Autodesk Fusion 360 part; units mm, degrees
sketch "Sketch1" plane through (0, 0, 0) normal (1, 0, 0) x (0, 1, 0)
  line L0 (0, 7) -> (2, 7)
  line L1 (2, 7) -> (2, 0)
  line L2 (0, 0) -> (0, 12.5)
  line L3 (0, 12.5) -> (-30.8, 12.5)
  line L4 (-30.8, 12.5) -> (-30.8, 0)
  line L5 (-30.8, 12.2) -> (-61.6, 12.2)
  line L6 (-61.6, 12.2) -> (-61.6, 0)
  line L7 (-61.6, 0) -> (0, 0)
  line L8 (2, 3) -> (15, 3)
  line L9 (15, 3) -> (15, 0)
  line L10 (15, 0) -> (0, 0)
  line L11 (-61.6, -12.2) -> (-61.6, 0)
  line L12 (-30.8, -12.2) -> (-61.6, -12.2)
  line L13 (-30.8, -12.5) -> (-30.8, 0)
  line L14 (0, -12.5) -> (-30.8, -12.5)
  line L15 (0, 0) -> (0, -12.5)
  line L16 (0, -7) -> (2, -7)
  line L17 (2, -7) -> (2, 0)
  line L18 (2, -3) -> (15, -3)
  line L19 (15, -3) -> (15, 0)
  dimension "d1" = 25
  dimension "d2" = 24.4
  dimension "d3" = 14
  dimension "d4" = 6
  dimension "d5" = 15
  dimension "d7" = 30.8
  dimension "d8" = 30.8
  dimension "d9" = 2
revolve "Revolve1" add sketch "Sketch1" angle 360 about axis through (0, 1.75, 0) along (0, 1, 0) contours L0 L1 L2 L10 | L2 L3 L4 L7 | L1 L8 L9 L10 | L4 L5 L6 L7
sketch "Sketch2" plane through (0, 15, 0) normal (0, 1, 0) x (-1, 0, 0)
  circle A0 centre (0, 0) radius 3
  circle A1 centre (0, 0) radius 3
  line L0 (-2.2361, 2) -> (2.2361, 2)
  line L1 (0, 0) -> (0, -3)
  point P0 (0, -3)
  dimension "d11" = 6
  dimension "d12" = 5
extrude "Extrude1" cut sketch "Sketch2" against normal blind 9 contours A0 A1 L0 picked at (-0.1433, 0.3437)
sketch "Sketch3" plane through (0, 0, 0) normal (0, 1, 0) x (-1, 0, 0)
  circle A0 centre (0, 0) radius 12.5
  circle A1 centre (0, 0) radius 7
  circle A2 centre (-6.8943, 6.8943) radius 1.5
  circle A3 centre (6.8943, 6.8943) radius 1.5
  circle A4 centre (6.8943, -6.8943) radius 1.5
  circle A5 centre (-6.8943, -6.8943) radius 1.5
  line L0 (0, 0) -> (-6.8943, 6.8943)
  line L1 (0, 0) -> (6.8943, 6.8943)
  line L2 (6.8943, -6.8943) -> (0, 0)
  line L3 (0, 0) -> (-6.8943, -6.8943)
  circle A6 centre (0, 0) radius 9.75
  line L4 (0, 0) -> (2.2693, 0)
  dimension "d15" = 3
  dimension "d16" = 19.5
  dimension "d20" = 45
extrude "Extrude2" cut sketch "Sketch3" against normal blind 4.6 contours A3 L1 A6 | A3 L1 A6 | A4 L2 A6 | A4 L2 A6 | A2 L0 A6 | A2 L0 A6 | A3 A6 | A5 L3 A6 | A5 L3 A6 | A4 A6 | A2 A6 | A5 A6
sketch "Sketch4" plane through (0, -61.6, 0) normal (0, -1, 0) x (1, 0, 0)
  circle A0 centre (0, 0) radius 12.2
  circle A1 centre (0, 0) radius 10
  dimension "d23" = 20
extrude "Extrude3" add sketch "Sketch4" along normal blind 5 contours A1
extrude "Extrude4" add 1 faces at (-0.4082, 15, 2.4414) along direction (0, 1, 0) blind 5
equation "d16 = 14 mm + ( ( 25 - 14 ) / 2 ) * 1 mm"
Build history of the part. All positions in model axes, mm. A direction names the side the tool comes from. Give positions to 0.01 mm unless a question says otherwise; leave off trailing zeros. Order: outer loops, then holes, each group sorted by start corner. A loop starts at its lowest first (then second) coordinate and runs counter-clockwise, first axis right, second up. Notation, with made-up numbers: M 78,28.5 L 134,28.5 A14 cw 134,39.5 Z; hole C 48.25,82.5 d4. An arc over 180 degrees is marked long. Put each result on its own line as item: value.
Item 1: Wall check: probe 1 along Y at (x, z) = (7.5, 6.75); probe 2 along Y at (x, z) = (1.5, 4.5); probe 3 along X at (y, z) = (-15, 0). Give the ranges that are in metal, low to high.
Results are:
probe 1: -61.6 to -4.6
probe 2: -66.6 to 2
probe 3: -12.5 to 12.5
Item 2: Cut at C-C on y = -35. Write the cut outline in (x, z), then the cut area to 3 significant figures.
Results are:
outline: C 0,0 d24.4
area: 468 mm2
Item 3: Which spindle directions (+Z, -Z, +X, -X, +Y, -Y) get a long thin tool onto all of the face, cutting with end or side? Do faces 1 (the face through (7, -4.6, -7)), 2 (the face through (-0.54, -46.42, -12.19)), 3 (the face through (0, 6, 0)). Say none if no direction does.
Results are:
face 1: +Y
face 2: -Y
face 3: -Z, +X, -X, +Y
Item 4: Drop flat-ended pins along their axis: pin 1 Ø2.5 at (x, z) = (1, 0) entering from +Y; pin 2 Ø10 at (y, z) = (7, 7.5) entering from -X; pin 3 Ø3.5 at (x, z) = (6.89, 6.89) entering from +Y. Give the stop position or say it passes through.
Results are:
pin 1: y = 6
pin 2: x = -1.66
pin 3: y = 0
Item 5: Pull direction Z, two halves, no side cores. Call faces 4 (the face through (-5.4, 0, 5.4)), 5 (the face through (8.1, -2.3, 6)), 6 (the face through (0, 13, 2)), 7 (the face through (-7, -4.6, -7)): +Z half, -Z half, draft (parallel to the pull), parting line (faces both ways), or undercut.
Results are:
face 4: draft
face 5: undercut
face 6: -Z half
face 7: undercut
Item 6: Cut at B-B on x = 0. Write the cut outline in (y, z), then the cut area to 3 significant figures.
Results are:
outline: M -66.6,-10 L -61.6,-10 L -61.6,-12.2 L -30.8,-12.2 L -30.8,-12.5 L 0,-12.5 L 0,-7 L 2,-7 L 2,-3 L 6,-3 L 6,2 L 20,2 L 20,3 L 2,3 L 2,7 L 0,7 L 0,12.5 L -30.8,12.5 L -30.8,12.2 L -61.6,12.2 L -61.6,10 L -66.6,10 Z
area: 1,690 mm2
Item 7: Cut at A-A on z = 0. Write the cut outline in (x, y).
Results are:
outline: M -12.5,-30.8 L -12.2,-30.8 L -12.2,-61.6 L -10,-61.6 L -10,-66.6 L 10,-66.6 L 10,-61.6 L 12.2,-61.6 L 12.2,-30.8 L 12.5,-30.8 L 12.5,0 L 7,0 L 7,2 L 3,2 L 3,6 L -3,6 L -3,2 L -7,2 L -7,0 L -12.5,0 Z
Item 8: Cut at D-D on y = -13.5. Write the cut outline in (x, z), then the cut area to 3 significant figures.
Results are:
outline: C 0,0 d25
area: 491 mm2
